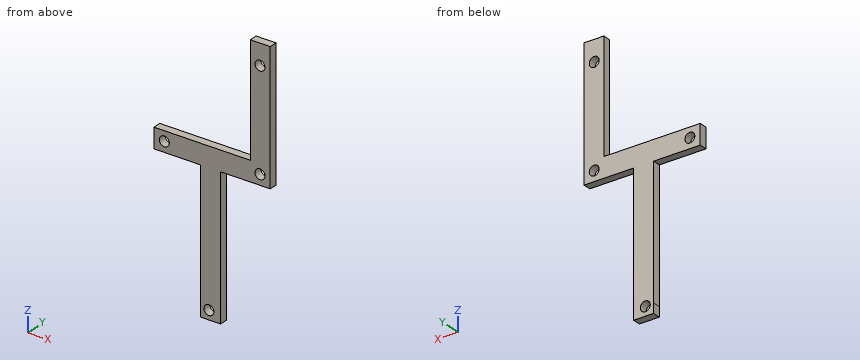
from build123d import *

# Parameters (mm, degrees)
SALIENTE_EXTRUIR2_DEPTH = 2
CROQUIS2_R              = 1.25
CORTAR_EXTRUIR1_DEPTH   = 2


with BuildPart() as part:
    # Croquis1 → Saliente-Extruir2 (new body)
    with BuildSketch(Plane(origin=(0, 0, 0), x_dir=(1, 0, 0), z_dir=(0, 1, 0))):
        Polygon((15.056023907, 39.704773072), (15.056023907, 26.168187684), (15.056023907, 7.074316274), (3.362466557, 7.074316274), (3.362466557, 2.074316274), (27.565385425, 2.074316274), (27.565385425, -25.657265495), (32.565385425, -25.657265495), (32.565385425, 7.074316274), (20.094799992, 7.074316274), (20.094799992, 42.092248366), (15.094799992, 42.092248366), align=None)
    extrude(amount=SALIENTE_EXTRUIR2_DEPTH)

    # Croquis2 → Cortar-Extruir1 (cut)
    with BuildSketch(Plane(origin=(0, 2, 0), x_dir=(1, 0, 0), z_dir=(0, 1, 0))):
        with Locations(Location((17.158653271, 39.819787948, 0), (0, 0, 270))):
            Circle(CROQUIS2_R)
        with Locations(Location((5.962263761, 4.535787948, 0), (0, 0, 270))):
            Circle(CROQUIS2_R)
        with Locations(Location((29.988653271, 4.535787948, 0), (0, 0, 270))):
            Circle(CROQUIS2_R)
        with Locations(Location((29.988653271, -20.46630955, 0), (0, 0, 270))):
            Circle(CROQUIS2_R)
    extrude(amount=-CORTAR_EXTRUIR1_DEPTH, mode=Mode.SUBTRACT)


solid = part.part
Source: CAD feature listing. Evaluate the final solid. Frame: model axes, mm. Round coordinates to 2 decimals unless told otherwise and drop trailing zeros. Loops run counter-clockwise (first coordinate to the right, second up) from the corner with the lowest first, then second, coordinate; pieces in that order, holes last.
Q1. First-contact query: P1, Ø0.6, axis at y = 1, z = -31, coming from the +X side; P2, Ø1, axis at y = 1.5, z = -16.5, coming from the -X side; P3, Ø0.6, axis at x = 15.5, y = 1, coming from the +Z side; P4, Ø2, axis at x = 17.16, z = -39.82, coming from the +Y side. Flat tips, straight axial feed; report the tip coordinate or a pass-through.
Q2. Section A-A, the plane y = 1.05. Return loops of the section in (x, z).
Q3. Section D-D, the plane z = -34. Return loops of the section in (x, y).
Q4. Section B-B, the plane z = -5. Return loops of the section in (x, y).
Q5. Section C-C, the plane x = 12.25. Return loops of the section in (y, z).
Q6. Ray query, line 1 (Z direction, x = 29.25, y = 1.25); line 2 (X direction, y = 0.8, z = 14.5); line 3 (X direction, y = 0.7, z = -35). Return the intervals inside material, ascending.
Solutions:
1. P1: stops at x = 20.09
1. P2: stops at x = 15.06
1. P3: stops at z = -2.07
1. P4: passes through
2. outline: (3.36, -7.07) - (15.06, -7.07) - (15.06, -39.7) - (15.09, -42.09) - (20.09, -42.09) - (20.09, -7.07) - (32.57, -7.07) - (32.57, 25.66) - (27.57, 25.66) - (27.57, -2.07) - (3.36, -2.07) - close; hole circle Ø2.5 at (5.96, -4.54); hole circle Ø2.5 at (17.16, -39.82); hole circle Ø2.5 at (29.99, -4.54); hole circle Ø2.5 at (29.99, 20.47)
3. outline: (15.06, 0) - (20.09, 0) - (20.09, 2) - (15.06, 2) - close
4. outline: (3.36, 0) - (4.8, 0) - (4.8, 2) - (3.36, 2) - close; (7.12, 0) - (28.83, 0) - (28.83, 2) - (7.12, 2) - close; (31.15, 0) - (32.57, 0) - (32.57, 2) - (31.15, 2) - close
5. outline: (0, -7.07) - (2, -7.07) - (2, -2.07) - (0, -2.07) - close
6. line 1: z = -7.07 to -5.54, -3.53 to 19.46, 21.47 to 25.66
6. line 2: x = 27.57 to 32.57
6. line 3: x = 15.06 to 20.09
